Can you work these out from the model? Positions are in its coordinate system, mm. Face numbers are marked on the shaded views. Round coordinates to 2 decimals unless told otherwise and drop trailing zeros. Order: outer loops, then holes, each group sorted by start corner. A loop starts at its lowest first (then second) coordinate and runs counter-clockwise, first axis right, second up.
Q1. If I drill on line 1 (Y direction, x = -6.5, z = 2.2); line 2 (X direction, y = 31.5, z = 3.8); line 3 (Y direction, x = 39, z = 0.7), over which ranges is the centre line in solid material (lowest first)?
Q2. If we section it at A-A (y = -10): Please give me the cut outline in (x, z).
Q3. We'd pull the mould along Y, two halves only. Please class the marked faces 1 and 2: pulls with the +Y half, pulls with the -Y half, needs draft (parallel to the pull), parting line crosses it, or undercut.
Q4. Will these pins go through, and if not, where does the flat tip stop? P1, Ø2.5, axis at y = 0, z = 3.5, coming from the -X side; P2, Ø1.7, axis at y = 4, z = 1.5, coming from the -X side; P3, Ø1, axis at x = -6, y = -5, coming from the +Z side.
Q5. If we section it at B-B (x = -11): Please give me the cut outline in (y, z).
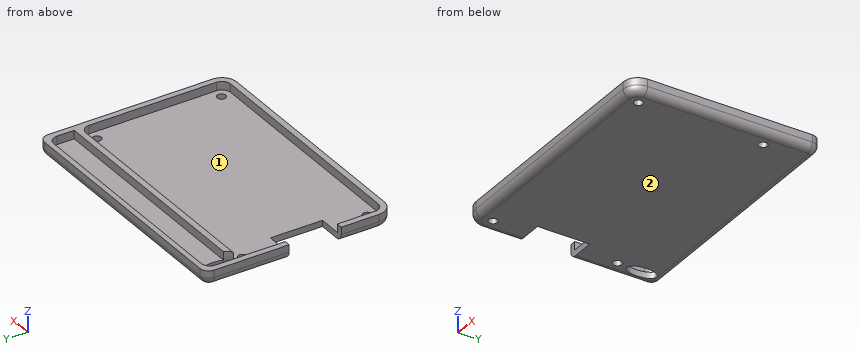
from build123d import *

# Parameters (mm, degrees)
F0_R     = 1.5
F1_DEPTH = 2.1
F2_DEPTH = 5
F3_R     = 2.5


with BuildPart() as f1:
    # F0 (on Top) → F1 (new body)
    with BuildSketch(Plane.XY):
        with BuildLine():
            Line((39.5, -25), (34.5, -25))
            Line((34.5, -25), (-34.5, -25))
            Line((-34.5, -25), (-39.5, -25))
            ThreePointArc((-39.5, -25), (-41.62132, -24.12132), (-42.5, -22))
            Line((-42.5, -22), (-42.5, -9))
            Line((-42.5, -9), (-44.6, -9))
            Line((-44.6, -9), (-44.6, -22))
            ThreePointArc((-44.6, -22), (-43.106245, -25.606245), (-39.5, -27.1))
            Line((-39.5, -27.1), (39.5, -27.1))
            ThreePointArc((39.5, -27.1), (43.106245, -25.606245), (44.6, -22))
            Line((44.6, -22), (44.6, 22))
            Line((44.6, 22), (44.6, 34.9))
            ThreePointArc((44.6, 34.9), (43.72132, 37.02132), (41.6, 37.9))
            Line((41.6, 37.9), (0, 37.9))
            Line((0, 37.9), (-41.6, 37.9))
            ThreePointArc((-41.6, 37.9), (-43.72132, 37.02132), (-44.6, 34.9))
            Line((-44.6, 34.9), (-44.6, 22))
            Line((-44.6, 22), (-44.6, 9))
            Line((-44.6, 9), (-42.5, 9))
            Line((-42.5, 9), (-42.5, 22))
            Line((-42.5, 22), (-42.5, 27.1))
            Line((-42.5, 27.1), (-42.5, 33.1))
            ThreePointArc((-42.5, 33.1), (-41.62132, 35.22132), (-39.5, 36.1))
            Line((-39.5, 36.1), (0, 36.1))
            Line((0, 36.1), (39.5, 36.1))
            ThreePointArc((39.5, 36.1), (41.62132, 35.22132), (42.5, 33.1))
            Line((42.5, 33.1), (42.5, 27.1))
            Line((42.5, 27.1), (42.5, 22))
            Line((42.5, 22), (42.5, -22))
            ThreePointArc((42.5, -22), (41.62132, -24.12132), (39.5, -25))
        make_face()
        with BuildLine():
            Line((-34.5, 9), (-34.5, 25))
            Line((-34.5, 25), (-39.461525, 25))
            add(Edge.make_bspline(
                [(-39.5, 25), (-39.480766, 24.999701), (-39.461525, 25)],
                knots=[0, 0, 0, 0.015266, 0.015266, 0.015266], degree=2, weights=[1, 0.999971, 1]))
            ThreePointArc((-39.5, 25), (-41.62132, 24.12132), (-42.5, 22))
            Line((-42.5, 22), (-42.5, 9))
            Line((-42.5, 9), (-34.5, 9))
        make_face()
        with Locations((-39, 21.5)):
            Circle(F0_R, mode=Mode.SUBTRACT)
        with BuildLine():
            Line((-34.5, -25), (-34.5, -9))
            Line((-34.5, -9), (-42.5, -9))
            Line((-42.5, -9), (-42.5, -22))
            ThreePointArc((-42.5, -22), (-41.62132, -24.12132), (-39.5, -25))
            Line((-39.5, -25), (-34.5, -25))
        make_face()
        with Locations((-39, -21.5)):
            Circle(F0_R, mode=Mode.SUBTRACT)
        Polygon((34.5, 25), (-34.5, 25), (-34.5, 9), (-34.5, -9), (-34.5, -25), (34.5, -25), align=None)
        with BuildLine():
            Line((39.5, 25), (34.5, 25))
            Line((34.5, 25), (34.5, -25))
            Line((34.5, -25), (39.5, -25))
            ThreePointArc((39.5, -25), (41.62132, -24.12132), (42.5, -22))
            Line((42.5, -22), (42.5, 22))
            ThreePointArc((42.5, 22), (41.62132, 24.12132), (39.5, 25))
        make_face()
        with Locations((39, -21.5)):
            Circle(F0_R, mode=Mode.SUBTRACT)
        with Locations((39, 21.5)):
            Circle(F0_R, mode=Mode.SUBTRACT)
        with BuildLine():
            ThreePointArc((-42.5, 22), (-41.62132, 24.12132), (-39.5, 25))
            add(Edge.make_bspline(
                [(-41.488852, 27.1), (-40.765333, 25.019686), (-39.5, 25)],
                knots=[5.35244, 5.35244, 5.35244, 6.283185, 6.283185, 6.283185], degree=2, weights=[1, 0.893654, 1]))
            Line((-41.488852, 27.1), (-42.5, 27.1))
            Line((-42.5, 27.1), (-42.5, 22))
        make_face()
        with BuildLine():
            add(Edge.make_bspline(
                [(-37.42306, 27.1), (-34.387845, 35.271957), (-39.359425, 35.271957), (-44.331004, 35.271957), (-41.488852, 27.1)],
                knots=[0.946012, 0.946012, 0.946012, 3.149226, 3.149226, 5.35244, 5.35244, 5.35244], degree=2, weights=[1, 0.452163, 1, 0.452163, 1]))
            Line((-37.42306, 27.1), (39.5, 27.1))
            Line((39.5, 27.1), (42.5, 27.1))
            Line((42.5, 27.1), (42.5, 33.1))
            ThreePointArc((42.5, 33.1), (41.62132, 35.22132), (39.5, 36.1))
            Line((39.5, 36.1), (0, 36.1))
            Line((0, 36.1), (-39.5, 36.1))
            ThreePointArc((-39.5, 36.1), (-41.62132, 35.22132), (-42.5, 33.1))
            Line((-42.5, 33.1), (-42.5, 27.1))
            Line((-42.5, 27.1), (-41.488852, 27.1))
        make_face()
        with BuildLine():
            Line((-39.461525, 25), (-34.5, 25))
            Line((-34.5, 25), (34.5, 25))
            Line((34.5, 25), (39.5, 25))
            ThreePointArc((39.5, 25), (41.62132, 24.12132), (42.5, 22))
            Line((42.5, 22), (42.5, 27.1))
            Line((42.5, 27.1), (39.5, 27.1))
            Line((39.5, 27.1), (-37.42306, 27.1))
            add(Edge.make_bspline(
                [(-39.461525, 25), (-38.195727, 25.019686), (-37.42306, 27.1)],
                knots=[0.015266, 0.015266, 0.015266, 0.946012, 0.946012, 0.946012], degree=2, weights=[1, 0.893654, 1]))
        make_face()
    extrude(amount=F1_DEPTH)

    # F0 (on Top) → F2 (join)
    with BuildSketch(Plane.XY):
        with BuildLine():
            Line((39.5, -25), (34.5, -25))
            Line((34.5, -25), (-34.5, -25))
            Line((-34.5, -25), (-39.5, -25))
            ThreePointArc((-39.5, -25), (-41.62132, -24.12132), (-42.5, -22))
            Line((-42.5, -22), (-42.5, -9))
            Line((-42.5, -9), (-44.6, -9))
            Line((-44.6, -9), (-44.6, -22))
            ThreePointArc((-44.6, -22), (-43.106245, -25.606245), (-39.5, -27.1))
            Line((-39.5, -27.1), (39.5, -27.1))
            ThreePointArc((39.5, -27.1), (43.106245, -25.606245), (44.6, -22))
            Line((44.6, -22), (44.6, 22))
            Line((44.6, 22), (44.6, 34.9))
            ThreePointArc((44.6, 34.9), (43.72132, 37.02132), (41.6, 37.9))
            Line((41.6, 37.9), (0, 37.9))
            Line((0, 37.9), (-41.6, 37.9))
            ThreePointArc((-41.6, 37.9), (-43.72132, 37.02132), (-44.6, 34.9))
            Line((-44.6, 34.9), (-44.6, 22))
            Line((-44.6, 22), (-44.6, 9))
            Line((-44.6, 9), (-42.5, 9))
            Line((-42.5, 9), (-42.5, 22))
            Line((-42.5, 22), (-42.5, 27.1))
            Line((-42.5, 27.1), (-42.5, 33.1))
            ThreePointArc((-42.5, 33.1), (-41.62132, 35.22132), (-39.5, 36.1))
            Line((-39.5, 36.1), (0, 36.1))
            Line((0, 36.1), (39.5, 36.1))
            ThreePointArc((39.5, 36.1), (41.62132, 35.22132), (42.5, 33.1))
            Line((42.5, 33.1), (42.5, 27.1))
            Line((42.5, 27.1), (42.5, 22))
            Line((42.5, 22), (42.5, -22))
            ThreePointArc((42.5, -22), (41.62132, -24.12132), (39.5, -25))
        make_face()
        with BuildLine():
            Line((-39.461525, 25), (-34.5, 25))
            Line((-34.5, 25), (34.5, 25))
            Line((34.5, 25), (39.5, 25))
            ThreePointArc((39.5, 25), (41.62132, 24.12132), (42.5, 22))
            Line((42.5, 22), (42.5, 27.1))
            Line((42.5, 27.1), (39.5, 27.1))
            Line((39.5, 27.1), (-37.42306, 27.1))
            add(Edge.make_bspline(
                [(-39.461525, 25), (-38.195727, 25.019686), (-37.42306, 27.1)],
                knots=[0.015266, 0.015266, 0.015266, 0.946012, 0.946012, 0.946012], degree=2, weights=[1, 0.893654, 1]))
        make_face()
    extrude(amount=F2_DEPTH)

    # F3
    f3_edges = [f1.edges().sort_by_distance(p)[0] for p in [
        (44.6, 6.45, 0),
    ]]
    fillet(f3_edges, radius=F3_R)


solid = f1.part
Solution:
1. line 1: y = -27.08 to -25, 25 to 27.1, 36.1 to 37.88
1. line 2: x = -44.6 to -42.5, 42.5 to 44.6
1. line 3: y = -26.33 to -23, -20 to 20, 23 to 37.13
2. outline: (-44.6, 2.5) arc R2.5 ccw to (-42.1, 0) - (42.1, 0) arc R2.5 ccw to (44.6, 2.5) - (44.6, 5) - (42.5, 5) - (42.5, 2.1) - (-42.5, 2.1) - (-42.5, 5) - (-44.6, 5) - close
3. face 1: undercut
3. face 2: needs draft
4. P1: stops at x = 42.5
4. P2: stops at x = -34.5
4. P3: stops at z = 2.1
5. outline: (-27.1, 2.5) arc R2.5 ccw to (-24.6, 0) - (35.4, 0) arc R2.5 ccw to (37.9, 2.5) - (37.9, 5) - (36.1, 5) - (36.1, 2.1) - (27.1, 2.1) - (27.1, 5) - (25, 5) - (25, 2.1) - (-25, 2.1) - (-25, 5) - (-27.1, 5) - close
